Input: part model. Units: mm. Frame: model coordinates. A direction names the side the tool comes from. Round coordinates to 2 decimals unless told otherwise and drop trailing zeros. Order: outer loops, then holes, each group sorted by start corner. A loop starts at its lowest first (then second) coordinate and runs counter-clockwise, first axis right, second up. Notation, with made-up numbers: (56.25, 12.5) -> (101.25, 12.5) arc R17 ccw to (101.25, 19.5) -> close; hole circle Ø4 at (24.25, 78). An arc over 180 degrees is marked (long way). Answer as CSV lines item,"result". Start each with the question number.
1) Section query A-A, the plane x = 57.5. Output: boundary loops of the cut face in (y, z).
2) Mould query, pull axis Z, two halves, no side actions, for faces 3 (the face through (-4, 10, -200)), 4 (the face through (-156, 10, -150)), 5 (the face through (-300, 10, 3)). Classes: +Z half, -Z half, draft (parallel to the pull), parting line (faces both ways), or undercut.
3) Section query B-B, the plane z = -84. Output: boundary loops of the cut face in (x, y), and give its area (3 significant figures).
4) Section query C-C, the plane y = 14. Output: boundary loops of the cut face in (x, z).
5) Line query: L1, parallel to X at y = 6.25, z = 48; L2, parallel to Z at x = 122, y = 4. Output: solid intervals per line, ascending.
6) Access query for faces 1 (the face through (300, 10, 3)), 2 (the face through (150, 10, 2)). Directions: +Z, -Z, +X, -X, +Y, -Y. A direction counts if a zero-diameter tool reaches every point of the face in a straight line with its end or side. Return the directions, or none.
```python
from build123d import *

# Parameters (mm, degrees)
SKETCH1_W           = 600
SKETCH1_H           = 400
BOSS_EXTRUDE2_DEPTH = 20
SKETCH1_10_W        = 190
SKETCH1_10_H        = 300
BOSS_EXTRUDE5_DEPTH = 20


with BuildPart() as part:
    # Sketch1 → Boss-Extrude2 (new body)
    with BuildSketch(Plane(origin=(0, 0, 0), x_dir=(1, 0, 0), z_dir=(0, 1, 0))):
        Rectangle(SKETCH1_W, SKETCH1_H)
        Polygon((170, -150), (170, 150), (170, 170), (-270, 170), (-270, -170), (170, -170), align=None, mode=Mode.SUBTRACT)
    extrude(amount=BOSS_EXTRUDE2_DEPTH)

    # Sketch1_10 → Boss-Extrude5 (add)
    with BuildSketch(Plane(origin=(0, 0, 0), x_dir=(1, 0, 0), z_dir=(0, 1, 0))):
        Polygon((170, -150), (170, -170), (-270, -170), (-270, 170), (170, 170), (170, 150), align=None)
        with Locations((55, 0)):
            Rectangle(SKETCH1_10_W, SKETCH1_10_H, mode=Mode.SUBTRACT)
        with Locations((-155, 0)):
            Rectangle(SKETCH1_10_W, SKETCH1_10_H, mode=Mode.SUBTRACT)
    extrude(amount=BOSS_EXTRUDE5_DEPTH)


solid = part.part
```
Findings:
1,outline,"(0, -200) -> (20, -200) -> (20, -150) -> (0, -150) -> close; (0, 150) -> (20, 150) -> (20, 200) -> (0, 200) -> close"
2,face 3,"-Z half"
2,face 4,"undercut"
2,face 5,"draft"
3,outline,"(-300, 0) -> (-250, 0) -> (-250, 20) -> (-300, 20) -> close; (-60, 0) -> (-40, 0) -> (-40, 20) -> (-60, 20) -> close; (150, 0) -> (300, 0) -> (300, 20) -> (150, 20) -> close"
3,area,"4,400 mm^2"
4,outline,"(-300, -200) -> (300, -200) -> (300, 200) -> (-300, 200) -> close; hole (-250, -150) -> (-60, -150) -> (-60, 150) -> (-250, 150) -> close; hole (-40, -150) -> (150, -150) -> (150, 150) -> (-40, 150) -> close"
5,L1,"x = -300 to -250, -60 to -40, 150 to 300"
5,L2,"z = -200 to -150, 150 to 200"
6,face 1,"+Z, -Z, +X, +Y, -Y"
6,face 2,"+Y, -Y"
